Could you check a few things on this drawing? It's one solid part, dimensions in mm from its lowest x, y, z. Round coordinates to 2 decimals unless told otherwise and drop trailing zeros. Write each loop counter-clockwise with the first axis right and the second up, starting at its lowest first coordinate (ties: lowest second). Pieces come first, ordered by that corner, then holes. Notation, with made-up numbers: (72, 71) - (100, 71) arc R25 ccw to (100, 84) - close; hole circle Ø4 at (45.25, 40). An arc over 180 degrees is marked (long way). Use one line per item in the form item = value. Start each with the question number.
1. I want a section at C-C, the plane x = 21. List the corners of the cut face in (y, z) for me.
2. I want a section at D-D, the plane y = 1.5. List the corners of the cut face in (x, z) for me, plus the area to 3 significant figures.
3. I want a section at A-A, the plane z = 0.3. List the corners of the cut face in (x, y) for me, plus the area to 3 significant figures.
4. If I drill on line 1 along Y through (x, z) = (21, 1.8); line 2 along X through (y, z) = (2.75, 1); line 3 along X through (y, z) = (5, 0.35), over which ranges is the centre line in solid material (lowest first)?
5. I want a section at B-B, the plane y = 6.5. List the corners of the cut face in (x, z) for me, plus the area to 3 significant figures.
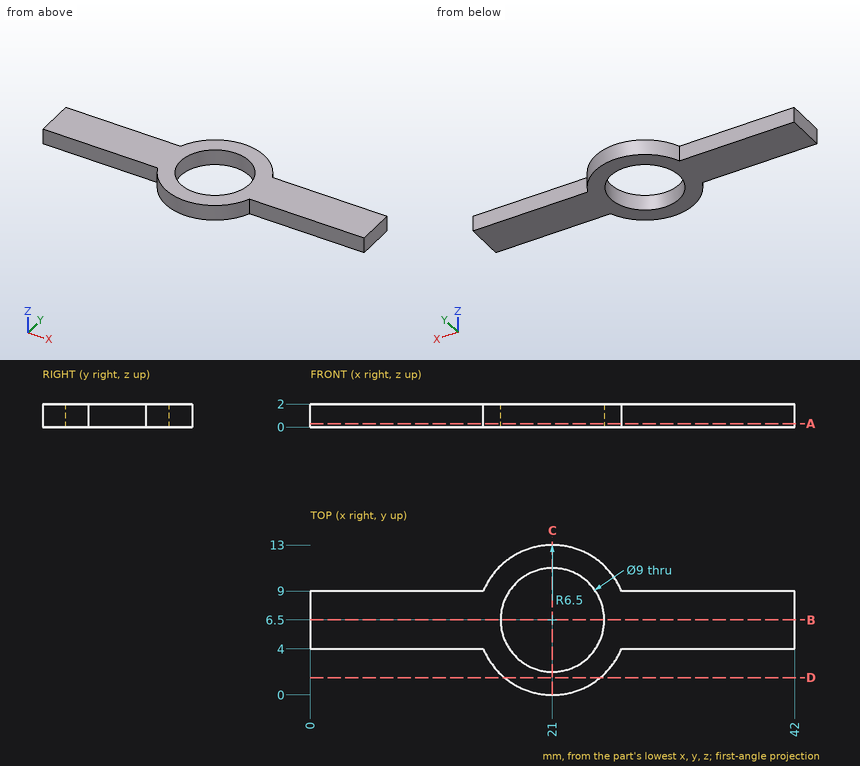
Model answer:
q1.outline = (0, 0) - (2, 0) - (2, 2) - (0, 2) - close; (11, 0) - (13, 0) - (13, 2) - (11, 2) - close
q2.outline = (16.85, 0) - (25.15, 0) - (25.15, 2) - (16.85, 2) - close
q2.area = 16.6 mm2
q3.outline = (0, 4) - (15, 4) arc R6.5 ccw to (27, 4) - (42, 4) - (42, 9) - (27, 9) arc R6.5 ccw to (15, 9) - (0, 9) - close; hole circle Ø9 at (21, 6.5)
q3.area = 216 mm2
q4.line_1 = 0 to 2, 11 to 13
q4.line_2 = 15.69 to 18.51, 23.49 to 26.31
q4.line_3 = 0 to 16.76, 25.24 to 42
q5.outline = (0, 0) - (16.5, 0) - (16.5, 2) - (0, 2) - close; (25.5, 0) - (42, 0) - (42, 2) - (25.5, 2) - close
q5.area = 66.0 mm2
